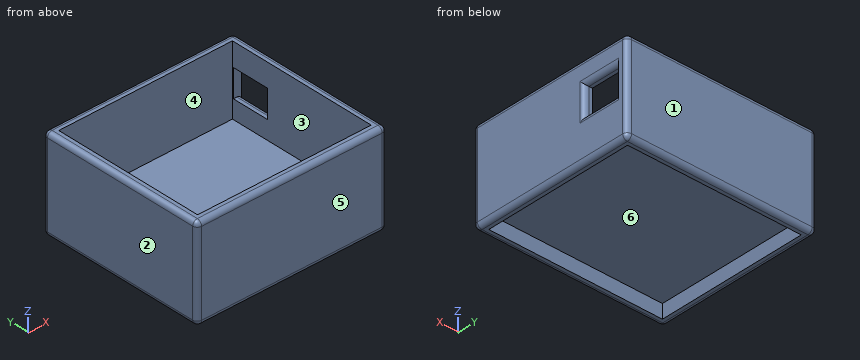
from build123d import *

# Parameters (mm, degrees)
SKETCH_W        = 41
SKETCH_H        = 36
PAD_DEPTH       = 20
SKETCH001_W     = 37.5
SKETCH001_H     = 32.5
POCKET_DEPTH    = 15
SKETCH002_W     = 37.5
SKETCH002_H     = 32.5
POCKET001_DEPTH = 3
SKETCH003_W     = 8
SKETCH003_H     = 6
POCKET002_DEPTH = 5
FILLET_R        = 1
FILLET001_R     = 1
FILLET002_R     = 1
FILLET003_R     = 1
FILLET004_R     = 1
FILLET005_R     = 1
FILLET006_R     = 1
FILLET007_R     = 1


with BuildPart() as part:
    # Sketch → Pad (new body)
    with BuildSketch(Plane.XY):
        Rectangle(SKETCH_W, SKETCH_H)
    extrude(amount=PAD_DEPTH)

    # Sketch001 (on Face6 of Pad) → Pocket (cut)
    with BuildSketch(Plane.XY.offset(20)):
        Rectangle(SKETCH001_W, SKETCH001_H)
    extrude(amount=-POCKET_DEPTH, mode=Mode.SUBTRACT)

    # Sketch002 (on Face4 of Pocket) → Pocket001 (cut)
    with BuildSketch(Plane(origin=(0, 0, 0), x_dir=(1, 0, 0), z_dir=(0, 0, -1))):
        Rectangle(SKETCH002_W, SKETCH002_H)
    extrude(amount=-POCKET001_DEPTH, mode=Mode.SUBTRACT)

    # Sketch003 (on Face3 of Pocket001) → Pocket002 (cut)
    with BuildSketch(Plane.YZ.offset(20.5)):
        with Locations((12, 12)):
            Rectangle(SKETCH003_W, SKETCH003_H)
    extrude(amount=-POCKET002_DEPTH, mode=Mode.SUBTRACT)

    # Fillet
    fillet_edges = [part.edges().sort_by_distance(p)[0] for p in [
        (-20.5, 0, 0),
    ]]
    fillet(fillet_edges, radius=FILLET_R)

    # Fillet001
    fillet001_edges = [part.edges().sort_by_distance(p)[0] for p in [
        (0.5, 18, 0),
    ]]
    fillet(fillet001_edges, radius=FILLET001_R)

    # Fillet002
    fillet002_edges = [part.edges().sort_by_distance(p)[0] for p in [
        (20.5, -0.5, 0),
    ]]
    fillet(fillet002_edges, radius=FILLET002_R)

    # Fillet003
    fillet003_edges = [part.edges().sort_by_distance(p)[0] for p in [
        (0, -18, 0),
    ]]
    fillet(fillet003_edges, radius=FILLET003_R)

    # Fillet004
    fillet004_edges = [part.edges().sort_by_distance(p)[0] for p in [
        (-20.5, 0, 20),
    ]]
    fillet(fillet004_edges, radius=FILLET004_R)

    # Fillet005
    fillet005_edges = [part.edges().sort_by_distance(p)[0] for p in [
        (20.5, 12, 9),
    ]]
    fillet(fillet005_edges, radius=FILLET005_R)

    # Fillet006
    fillet006_edges = [part.edges().sort_by_distance(p)[0] for p in [
        (20.5, 8, 12),
    ]]
    fillet(fillet006_edges, radius=FILLET006_R)

    # Fillet007
    fillet007_edges = [part.edges().sort_by_distance(p)[0] for p in [
        (20.5, 12, 15),
    ]]
    fillet(fillet007_edges, radius=FILLET007_R)


solid = part.part
The model under review builds one solid part; all positions refer to its coordinate system, in mm. Face numbers are marked on the shaded views. A direction names the side the tool comes from. Give positions to 0.01 mm unless a question says otherwise; leave off trailing zeros. Loops run counter-clockwise (first coordinate to the right, second up) from the corner with the lowest first, then second, coordinate; pieces in that order, holes last. Notation, with made-up numbers: (42.25, 8) -> (77.25, 8) arc R14 cw to (77.25, 21) -> close; hole circle Ø4 at (51, 48.25). An arc over 180 degrees is marked (long way). Write each question's results on one line, items separated by ' | '.
1) Draft analysis for pull direction Y (two halves, no side actions). For the marked faces 1, 2 and 3, state which applies: pulls with the +Y half, pulls with the -Y half, needs draft (parallel to the pull), parting line crosses it, or undercut.
Conclusion:
face 1: pulls with the +Y half | face 2: needs draft | face 3: undercut
2) Take a section at D-D, the plane y = 3. Give the boundary of the cut face in (x, z).
Conclusion:
outline: (-20.5, 1) arc R1 ccw to (-19.5, 0) -> (-18.75, 0) -> (-18.75, 3) -> (18.75, 3) -> (18.75, 0) -> (19.5, 0) arc R1 ccw to (20.5, 1) -> (20.5, 19) arc R1 ccw to (19.5, 20) -> (18.75, 20) -> (18.75, 5) -> (-18.75, 5) -> (-18.75, 20) -> (-19.5, 20) arc R1 ccw to (-20.5, 19) -> close
3) Insertion check: pin 1 Ø1 at (x, y) = (5, 5) entering from -Z; pin 2 Ø16 at (x, y) = (-1.5, 5.5) entering from +Z. Each pin has a flat end and moves straight along its axis. Give the tip position at first contact, or say it passes through.
Conclusion:
pin 1: stops at z = 3 | pin 2: stops at z = 5
4) Take a section at A-A, the plane y = 9. Give the boundary of the cut face in (x, z).
Conclusion:
outline: (-20.5, 1) arc R1 ccw to (-19.5, 0) -> (-18.75, 0) -> (-18.75, 3) -> (18.75, 3) -> (18.75, 0) -> (19.5, 0) arc R1 ccw to (20.5, 1) -> (20.5, 8) arc R1 ccw to (19.5, 9) -> (18.75, 9) -> (18.75, 5) -> (-18.75, 5) -> (-18.75, 20) -> (-19.5, 20) arc R1 ccw to (-20.5, 19) -> close; (18.75, 15) -> (19.5, 15) arc R1 ccw to (20.5, 16) -> (20.5, 19) arc R1 ccw to (19.5, 20) -> (18.75, 20) -> close
5) Take a section at B-B, the plane z = 18.5. Give the boundary of the cut face in (x, y), plus the area to 3 significant figures.
Conclusion:
outline: (-20.5, -17) arc R1 ccw to (-19.5, -18) -> (19.5, -18) arc R1 ccw to (20.5, -17) -> (20.5, 17) arc R1 ccw to (19.5, 18) -> (-19.5, 18) arc R1 ccw to (-20.5, 17) -> close; hole (-18.75, -16.25) -> (18.75, -16.25) -> (18.75, 16.25) -> (-18.75, 16.25) -> close | area: 256 mm^2
6) Tool access review of the marked faces 4, 5 and 6: name each direction out of +Z, -Z, +X, -X, +Y, -Y from which nothing blocks a thin tool from reaching the whole face with its end or side.
Conclusion:
face 4: +Z | face 5: +Z, -Z, +X, -X, -Y | face 6: -Z
7) Take a section at C-C, the plane x = 1.5. Give the boundary of the cut face in (y, z).
Conclusion:
outline: (-18, 1) arc R1 ccw to (-17, 0) -> (-16.25, 0) -> (-16.25, 3) -> (16.25, 3) -> (16.25, 0) -> (17, 0) arc R1 ccw to (18, 1) -> (18, 19) arc R1 ccw to (17, 20) -> (16.25, 20) -> (16.25, 5) -> (-16.25, 5) -> (-16.25, 20) -> (-17, 20) arc R1 ccw to (-18, 19) -> close
8) For line 1 along X through (y, z) = (-15, 12.75); line 2 along Y through (x, z) = (9, 19); line 3 along Z through (x, y) = (-12, -8), list the stretches that pass through material, from the lowest coordinate up. Write a range as from..to.
Conclusion:
line 1: x = -20.5..-18.75, 18.75..20.5 | line 2: y = -18..-16.25, 16.25..18 | line 3: z = 3..5
